Autodesk Inventor part; units mm, degrees
ref_plane "Work Plane1" through (0, 6.731, 0) normal (0, -1, 0) x (1, 0, 0)
ref_plane "Work Plane2" through (0, 0, -4.9911) normal (0, 0, 1) x (1, 0, 0)
ref_plane "YZ Plane" through (0, 0, 0) normal (1, 0, 0) x (0, 1, 0)
sketch "Sketch1" plane through (0, 0, 0) normal (0, 1, 0) x (-1, 0, 0)
  circle A0 centre (0, 0) radius 4.9911
  dimension "d0" = 9.9822
extrude "Extrusion1" add sketch "Sketch1" along normal blind 1.524
sketch "Sketch2" plane through (0, 1.524, 0) normal (0, 1, 0) x (1, 0, 0)
  point P0 (0, 0)
ref_plane "Work Plane1" through (0, 6.731, 0) normal (0, -1, 0) x (1, 0, 0)
sketch "Sketch3" plane through (0, 6.731, 0) normal (0, -1, 0) x (1, 0, 0)
  circle A0 centre (0, 0) radius 4.1593
  circle A1 centre (0, 0) radius 2.6035
  dimension "d4" = 8.3185
  dimension "d9" = 5.207
loft "Loft1" add profiles "Sketch3" section 1 edges at (4.9911, 1.524, 0) contours A0 | A1
hole "Hole1" at (0, 6.731, 0) direction (0, -1, 0) diameter 4.2418 end through all
extrude "Extrusion3" cut sketch "Sketch3" along normal blind 1.778 contours A1
ref_plane "Work Plane2" through (0, 0, -4.9911) normal (0, 0, 1) x (1, 0, 0)
chamfer "Chamfer1" distance 0.254 angle 45 1 edges at (4.9911, 0, 0)
sketch "Sketch4" plane through (0, 0, -4.9911) normal (0, 0, 1) x (1, 0, 0)
  line L0 (4.9911, 1.524) -> (-4.9911, 1.524)
  line L1 (0, 1.524) -> (0, 0)
  line L2 (2.5082, 1.524) -> (-2.5083, 1.524)
  line L3 (-2.5083, 1.524) -> (-2.5083, 0)
  line L4 (-2.5083, 0) -> (2.5082, 0)
  line L5 (2.5082, 0) -> (2.5082, 1.524)
  line L6 (2.5082, 1.524) -> (-2.5083, 0) construction
  line L7 (-2.5083, 1.524) -> (2.5082, 0) construction
  line L8 (2.9845, 1.524) -> (-2.9845, 1.524)
  line L9 (-2.9845, 1.524) -> (-2.9845, 0)
  line L10 (-2.9845, 0) -> (2.9845, 0)
  line L11 (2.9845, 0) -> (2.9845, 1.524)
  line L12 (2.9845, 1.524) -> (-2.9845, 0) construction
  line L13 (-2.9845, 1.524) -> (2.9845, 0) construction
  line L14 (2.9845, 1.524) -> (2.5082, 0)
  line L15 (-2.9845, 1.524) -> (-2.5083, 0)
  point P0 (4.9911, 0)
  point P1 (-4.9911, 0)
  point P2 (0, 0.762)
  dimension "d23" = 5.0165
  dimension "d24" = 5.969
extrude "Extrusion4" cut sketch "Sketch4" along normal through all contours L14 L5 L0 | L5 L4 L1 L0 | L1 L4 L3 L0 | L3 L15 L0
properties part number "0.375 Shaft Dovetail" material "Stainless Steel"
Could you check a few things on this model? Use its own coordinates, in mm. A direction names the side the tool comes from. Coordinates: 2 decimals unless noted, no trailing zeros. Write each loop counter-clockwise with the first axis right and the second up, starting at its lowest first coordinate (ties: lowest second). Pieces come first, ordered by that corner, then holes. Notation, with made-up numbers: (-27.5, -33) -> (5.5, -33) arc R20 ccw to (5.5, -17) -> close; hole circle Ø7 at (66, 81). An arc over 180 degrees is marked (long way). Write item = value, one per line. Start each with the question number.
(1) I need wall thicknesses on line 1 (Y direction, x = -0.25, z = -4); line 2 (X direction, y = 5.5, z = 1.25); line 3 (Z direction, x = 0, y = 5.9). Which ranges of each line are inside material? Lowest first, please. Write a range as [from, to].
(2) Will these pins go through, and if not, where does the flat tip stop? pin 1 (4 mm diameter, centred on y = 2, z = -1, fed in from -X); pin 2 (2 mm diameter, centred on y = 5, z = 2, fed in from -X); pin 3 (4.5 mm diameter, centred on x = 0, z = 0, fed in from -Y); pin 4 (3 mm diameter, centred on x = -2, y = 6, fed in from -Z).
(3) I want a section at A-A (x = 0). Please give me the cut outline in (y, z).
(4) Which directions (+Z, -Z, +X, -X, +Y, -Y) give clear straight access to the entire face, cutting with the end or side of a thin tool? Please do faces 1 (the face through (1.291, 3.214, -1.683)), 2 (the face through (0, 1.524, -2.3)).
(5) I want a section at B-B (y = 1). Please give me the cut outline in (x, z), plus the area to 3 significant figures.
(6) We'd pull the mould along Z, two halves only. Please class faces 3 (the face through (-4.865, 0.129, -0.07)), 4 (the face through (2.75, 0.77, -0.06)), 5 (the face through (2.483, 5.854, -0.782)): released by +Z, released by -Z, zero draft, split by the parting line, or undercut.
Result set:
q1.line_1 = [1.52, 6.73]
q1.line_2 = [-4.17, -2.28], [2.28, 4.17]
q1.line_3 = [-4.29, -2.6], [2.6, 4.29]
q2.pin_1 = -4.99
q2.pin_2 = -4.37
q2.pin_3 = 1.52
q2.pin_4 = -4.35
q3.outline = (1.52, -4.99) -> (6.73, -4.16) -> (6.73, -2.6) -> (4.95, -2.6) -> (4.95, -2.12) -> (1.52, -2.12) -> close; (1.52, 2.12) -> (4.95, 2.12) -> (4.95, 2.6) -> (6.73, 2.6) -> (6.73, 4.16) -> (1.52, 4.99) -> close
q4.face_1 = +Y, -Y
q4.face_2 = +Z, -Z
q5.outline = (-2.82, -4.12) -> (-2.82, 4.12) arc R4.99 ccw to start; (2.82, -4.12) arc R4.99 ccw to (2.82, 4.12) -> close
q5.area = 25.1 mm2
q6.face_3 = split by the parting line
q6.face_4 = zero draft
q6.face_5 = undercut
